Here's how the part is built. I have some questions about the finished solid (model axes, mm). A direction names the side the tool comes from. Round coordinates to 2 decimals unless told otherwise and drop trailing zeros. Order: outer loops, then holes, each group sorted by start corner. A loop starts at its lowest first (then second) coordinate and runs counter-clockwise, first axis right, second up. Notation, with made-up numbers: (73.5, 82) - (112.5, 82) arc R14 cw to (112.5, 98) - close; hole circle Ø10 at (31.25, 77.25). An arc over 180 degrees is marked (long way). Answer as a JSON object with one key per item and string values.
```python
from build123d import *

# Parameters (mm, degrees)
BOSS_EXTRUDE1_DEPTH = 106.5
TAP1_D              = 4.134
TAP1_DEPTH          = 12.4
TAP1_TIP            = 1.2419789
TAP2_D              = 4.134
TAP2_DEPTH          = 12.4
TAP2_TIP            = 1.2419789


with BuildPart() as part:
    # Sketch1 → Boss-Extrude1 (new body)
    with BuildSketch(Plane(origin=(0, 0, 0), x_dir=(0, 0, -1), z_dir=(1, 0, 0))):
        Polygon((0, -4.618802154), (4, -2.309401077), (4, 2.309401077), (0, 4.618802154), (-4, 2.309401077), (-4, -2.309401077), align=None)
    extrude(amount=BOSS_EXTRUDE1_DEPTH)

    # Sketch2 → Cut-Revolve1 (revolve, cut)
    with BuildSketch(Plane.XY):
        Polygon((0, 4.618802154), (0.35726559, 4.618802154), (0, 4), align=None)
        Polygon((106.14273441, 4.618802154), (106.5, 4), (106.5, 4.618802154), align=None)
    revolve(axis=Axis((0, 0, 0), (1, 0, 0)), mode=Mode.SUBTRACT)

    # Tap1
    with Locations(Plane.ZY):
        with Locations((0, 0)):
            Hole(TAP1_D / 2, depth=TAP1_DEPTH)
            with Locations((0, 0, -(TAP1_DEPTH + TAP1_TIP / 2))):  # 118° drill point
                Cone(0, TAP1_D / 2, TAP1_TIP, mode=Mode.SUBTRACT)

    # Tap2
    with Locations(Plane(origin=(106.5, 0, 0), x_dir=(0, 0, -1), z_dir=(1, 0, 0))):
        with Locations((0, 0)):
            Hole(TAP2_D / 2, depth=TAP2_DEPTH)
            with Locations((0, 0, -(TAP2_DEPTH + TAP2_TIP / 2))):  # 118° drill point
                Cone(0, TAP2_D / 2, TAP2_TIP, mode=Mode.SUBTRACT)


solid = part.part
```
1. If I drill on L1, parallel to Z at x = 101, y = 0; L2, parallel to Y at x = 9.5, z = 0; L3, parallel to X at y = -4, z = 0.5, over which ranges is the centre line in solid material (lowest first)? Write a range as [from, to].
Responses:
{"L1": "[-4, -2.07], [2.07, 4]", "L2": "[-4.62, -2.07], [2.07, 4.62]", "L3": "[0.02, 106.48]"}
2. For P1, Ø3.5, axis at y = 0, z = 0, coming from the +X side; P2, Ø2, axis at x = 67.5, z = 1.5, coming from the -Y side, each with a flat end and sliding along its axis, tell me the tip position at first contact or that it passes through.
Responses:
{"P1": "x = 93.91", "P2": "y = -4.33"}
3. Imagine slicing it at A-A (x = 10). List the corners of the cut face in (y, z) for me, plus the area to 3 significant figures.
Responses:
{"outline": "(-4.62, 0) - (-2.31, -4) - (2.31, -4) - (4.62, 0) - (2.31, 4) - (-2.31, 4) - close; hole circle Ø4.13 at (0, 0)", "area": "42.0 mm2"}
4. For faces 1 (the face through (52.5, 3.48, 1.97)), 2 (the face through (6.29, -1.26, 1.64)), which set-ups out of +Z, -Z, +X, -X, +Y, -Y let a thin tool reach every point of the face, with its end or its side?
Responses:
{"face 1": "+Z, +X, -X, +Y", "face 2": "-X"}
5. Imagine slicing it at B-B (x = 32). List the corners of the cut face in (y, z) for me.
Responses:
{"outline": "(-4.62, 0) - (-2.31, -4) - (2.31, -4) - (4.62, 0) - (2.31, 4) - (-2.31, 4) - close"}
6. Thinking about a two-plate mould opening in Y: for faces 3 (the face through (0.085, 2.065, -3.597)), 4 (the face through (52.505, -3.448, 2.028)), 5 (the face through (106.5, -2, -2)), 6 (the face through (100.21, -1.26, -1.64)), which applies, pulls with the +Y half, pulls with the -Y half, needs draft (parallel to the pull), parting line crosses it, or undercut?
Responses:
{"face 3": "pulls with the +Y half", "face 4": "pulls with the -Y half", "face 5": "needs draft", "face 6": "undercut"}
